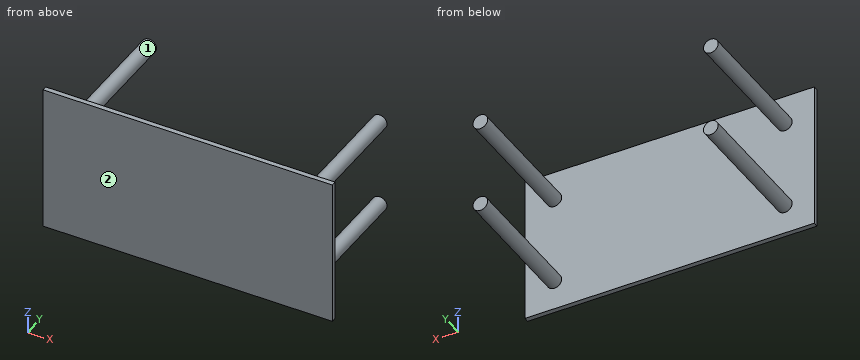
```python
from build123d import *

# Parameters (mm, degrees)
F0_W     = 59
F0_H     = 30
F1_DEPTH = 1
F2_R     = 1.5
F3_DEPTH = 27


with BuildPart() as f1:
    # F0 (on Front) → F1 (new body)
    with BuildSketch(Plane.XZ):
        Rectangle(F0_W, F0_H)
    extrude(amount=F1_DEPTH)

    # F2 (on face) → F3 (join)
    with BuildSketch(Plane(origin=(0, 0, 0), x_dir=(-1, 0, 0), z_dir=(0, 1, 0))):
        with Locations((23.5, 9)):
            Circle(F2_R)
        with Locations((-23.5, 9)):
            Circle(F2_R)
        with Locations((-23.5, -9)):
            Circle(F2_R)
        with Locations((23.5, -9)):
            Circle(F2_R)
    extrude(amount=F3_DEPTH)


solid = f1.part
```
Read the model definition and answer for the solid it produces. Units are mm, in the model's axes. Face numbers are marked on the shaded views. Coordinates: 2 decimals unless noted, no trailing zeros. Loops run counter-clockwise (first coordinate to the right, second up) from the corner with the lowest first, then second, coordinate; pieces in that order, holes last.
(1) Flat-ended cylindrical pins translate along their axes: pin 1 Ø1.5 at (y, z) = (12.5, 9) entering from -X; pin 2 Ø5 at (x, z) = (5.5, -8) entering from +Y; pin 3 Ø5 at (y, z) = (18, 7.5) entering from +X. Find the tip coordinate at first contact, or state that the pin passes through.
Solution:
pin 1: stops at x = -25
pin 2: stops at y = 0
pin 3: stops at x = 25
(2) The part is cut by section A-A (x = -23.5). Determine the outline of the cut face in (y, z), and give its area (3 significant figures).
Solution:
outline: (-1, -15) - (0, -15) - (0, -10.5) - (27, -10.5) - (27, -7.5) - (0, -7.5) - (0, 7.5) - (27, 7.5) - (27, 10.5) - (0, 10.5) - (0, 15) - (-1, 15) - close
area: 192 mm2
(3) Consider line 1 along Z through (x, y) = (-23.5, 23.5); line 2 along Y through (x, z) = (-6, 3); line 3 along X through (y, z) = (10.75, -10). Determine where each line is inside the solid, lowest interval first.
Solution:
line 1: z = -10.5 to -7.5, 7.5 to 10.5
line 2: y = -1 to 0
line 3: x = -24.62 to -22.38, 22.38 to 24.62
(4) The mould has two halves that part along X. Classify the marked faces 1 and 2: released by +X, released by -X, zero draft, split by the parting line, or undercut.
Solution:
face 1: undercut
face 2: zero draft
(5) The part is cut by section B-B (y = 12). Determine the outline of the cut face in (x, z).
Solution:
outline: circle Ø3 at (-23.5, -9); circle Ø3 at (-23.5, 9); circle Ø3 at (23.5, -9); circle Ø3 at (23.5, 9)
(6) The part is cut by section D-D (x = -17). Determine the outline of the cut face in (y, z).
Solution:
outline: (-1, -15) - (0, -15) - (0, 15) - (-1, 15) - close
(7) The part is cut by section C-C (z = 6.75). Determine the outline of the cut face in (x, y).
Solution:
outline: (-29.5, -1) - (29.5, -1) - (29.5, 0) - (-29.5, 0) - close
